Autodesk Inventor part; units mm, degrees
ref_plane "YZ Plane" through (0, 0, 0) normal (1, 0, 0) x (0, 1, 0)
ref_plane "XZ Plane" through (0, 0, 0) normal (0, 1, 0) x (-1, 0, 0)
ref_plane "XY Plane" through (0, 0, 0) normal (0, 0, 1) x (1, 0, 0)
sketch "Sketch1" plane through (0, 0, 0) normal (0, 0, 1) x (1, 0, 0)
  arc A0 (-6, 0) -> (6, 0) centre (0, 0) ccw
  arc A1 (0, -8) -> (8, 0) centre (0, 0) ccw
  line L0 (-6, -14) -> (-6, -50)
  line L1 (-8, 0) -> (-8, -50)
  line L2 (-6, 0) -> (-6, 20)
  line L3 (-8, 0) -> (-8, 20)
  line L4 (6, 0) -> (6, 20)
  line L5 (8, 0) -> (8, 20)
  line L6 (-8, -50) -> (-6, -50)
  line L7 (26.4346, -8) -> (-30.23, -8) construction
  arc A2 (0, -8) -> (-6, -14) centre (0, -14) ccw
  line L8 (8, 20) -> (6, 20)
  line L9 (-6, 20) -> (-8, 20)
  arc A3 (6, 0) -> (-6, 0) centre (0, 0) ccw construction
  dimension "d0" = 12
  dimension "d1" = 2
  dimension "d2" = 42
  dimension "d3" = 20
  dimension "d4" = 20
extrude "Højde" add sketch "Sketch1" along normal blind 16
sketch "Sketch3" plane through (-8, -50, 0) normal (-1, 0, 0) x (0, 0, 1)
  line L0 (0, 0) -> (0, 70)
  line L1 (0, 0) -> (16, 0)
  line L2 (16, 70) -> (16, 0)
  line L3 (0, 70) -> (16, 70)
  line L4 (0, 42) -> (16, 42)
  circle A0 centre (14, 24.5) radius 1.5
  circle A1 centre (14, 5.5) radius 1.5
  line L5 (18.141, 23) -> (9.2635, 23) construction
  line L6 (18.6037, 7) -> (9.7262, 7) construction
  line L7 (14, 3.0673) -> (14, 29.9023) construction
  line L8 (17.9327, 26) -> (8.2455, 26) construction
  line L9 (10.6205, 4) -> (2.6453, 4) construction
  circle A2 centre (8, 63) radius 2
  line L10 (16, 54) -> (0, 54) construction
  point P0 (0, 50)
  dimension "d7" = 3
  dimension "d8" = 3
  dimension "d9" = 16
  dimension "d10" = 22
  dimension "d11" = 4
  dimension "d12" = 16
  dimension "d13" = 14
  dimension "d14" = 4
  dimension "d15" = 7
  dimension "d16" = 8
  dimension "d17" = 12
extrude "Monteringshuller" cut sketch "Sketch3" against normal up to surface (16 mm away) contours A0 | A1 | A2
fillet "Fillet1" radius 1 17 edges at (8, 20, 8) (6, 20, 8) (-6, 20, 8) (-8, 20, 8) (-6, -50, 8) (-8, -50, 8) (-4.2426, -9.7574, 16) (5.6569, -5.6569, 16) (8, 10, 16) (-6, -32, 16) (-6, 10, 16) (6, 10, 16) (0, -6, 16) (-8, -15, 16) (-7, -50, 16) (7, 20, 16) (-7, 20, 16)
equation "\"d8\" = d7"
equation "\"d16\" = 0.5 * d12"
properties part number "Ø12-Z Endstop Holder"
Geometry check sheet. Reference: the model listing, model coordinates, mm. A direction names the side the tool comes from. Coordinates: 2 decimals unless noted, no trailing zeros. Answer as a JSON object with one key per item and string values.
1. Section check A-A, the plane z = 8. Give the number of separate pieces and of enclosed holes in the cut face, plus the area to 3 significant figures.
Answers below:
{"separate pieces": "3", "enclosed holes": "0", "area": "212 mm²"}
2. Draft check along X on faces 3 (the flat face through (-6, 9, 7)), 4 (the flat face through (-8, -15, 7)), 5 (the flat face through (-6, -31, 7)). Enter one of: released by +X, released by -X, zero draft, split by the parting line, or undercut.
Answers below:
{"face 3": "undercut", "face 4": "released by -X", "face 5": "released by +X"}
3. Scan lines: L1, parallel to Y at x = -6.95, z = 14; L2, parallel to X at y = 5, z = 10; L3, parallel to X at y = -33.5, z = 2. Record each from-to range of solid material in increasing order.
Answers below:
{"L1": "y = -50 to -46, -43 to -27, -24 to 20", "L2": "x = -8 to -6, 6 to 8", "L3": "x = -8 to -6"}
4. Tool access check on faces 1 (the flat face through (6, 9, 7)), 2 (the flat face through (-4, -7, 0)). Record the directions out of +Z, -Z, +X, -X, +Y, -Y that give a thin tool (end or side, any length) a straight path to the whole face; none if there is none.
Answers below:
{"face 1": "+Z, -Z, +Y", "face 2": "-Z, +X, -X, +Y, -Y"}
5. Go/stop test with flat-tipped pins: pin 1 Ø4.5 at (y, z) = (-34, 8) entering from +X; pin 2 Ø5 at (x, z) = (4, 11.5) entering from -Y; pin 3 Ø2 at (x, z) = (-1, 13.5) entering from -Y. Record where each tip stops, or that it passes through.
Answers below:
{"pin 1": "stops at x = -6", "pin 2": "stops at y = -7.86", "pin 3": "stops at y = -8.34"}
